Check sheet for the modelled part. Datum: model origin and axes. Units: mm. Round coordinates to 2 decimals unless told otherwise and drop trailing zeros. Write each loop counter-clockwise with the first axis right and the second up, starting at its lowest first coordinate (ties: lowest second). Pieces come first, ordered by that corner, then holes. Notation, with made-up numbers: (39, 74) -> (55, 74) arc R32 cw to (55, 109) -> close; hole circle Ø10 at (44, -31). An arc over 180 degrees is marked (long way). One line per item, written item: value.
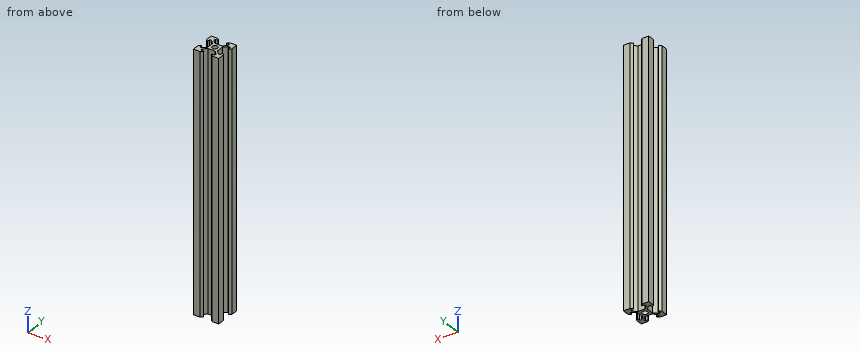
from build123d import *

# Parameters (mm, degrees)
SKETCH1_R           = 2.1
BOSS_EXTRUDE1_DEPTH = 200


with BuildPart() as part:
    # Sketch1 → Boss-Extrude1 (new body)
    with BuildSketch(Plane.XY):
        with BuildLine():
            Line((-2.839339828, 3.9), (-5.470710678, 6.53137085))
            ThreePointArc((-5.470710678, 6.53137085), (-5.492387953, 6.563813185), (-5.5, 6.602081528))
            Line((-5.5, 6.602081528), (-5.5, 8.1))
            ThreePointArc((-5.5, 8.1), (-5.470710678, 8.170710678), (-5.4, 8.2))
            Line((-5.4, 8.2), (-3.334418044, 8.2))
            ThreePointArc((-3.334418044, 8.2), (-3.244178397, 8.256909326), (-3.2566483, 8.362863876))
            Line((-3.2566483, 8.362863876), (-4.58, 10))
            Line((-4.58, 10), (-10, 10))
            Line((-10, 10), (-10, 4.58))
            Line((-10, 4.58), (-8.362863876, 3.2566483))
            ThreePointArc((-8.362863876, 3.2566483), (-8.256909326, 3.244178397), (-8.2, 3.334418044))
            Line((-8.2, 3.334418044), (-8.2, 5.4))
            ThreePointArc((-8.2, 5.4), (-8.170710678, 5.470710678), (-8.1, 5.5))
            Line((-8.1, 5.5), (-6.602081528, 5.5))
            ThreePointArc((-6.602081528, 5.5), (-6.563813185, 5.492387953), (-6.53137085, 5.470710678))
            Line((-6.53137085, 5.470710678), (-3.9, 2.839339828))
            Line((-3.9, 2.839339828), (-3.9, -2.839339828))
            Line((-3.9, -2.839339828), (-6.53137085, -5.470710678))
            ThreePointArc((-6.53137085, -5.470710678), (-6.563813185, -5.492387953), (-6.602081528, -5.5))
            Line((-6.602081528, -5.5), (-8.1, -5.5))
            ThreePointArc((-8.1, -5.5), (-8.170710678, -5.470710678), (-8.2, -5.4))
            Line((-8.2, -5.4), (-8.2, -3.334418044))
            ThreePointArc((-8.2, -3.334418044), (-8.256909326, -3.244178397), (-8.362863876, -3.2566483))
            Line((-8.362863876, -3.2566483), (-10, -4.58))
            Line((-10, -4.58), (-10, -10))
            Line((-10, -10), (-4.58, -10))
            Line((-4.58, -10), (-3.2566483, -8.362863876))
            ThreePointArc((-3.2566483, -8.362863876), (-3.244178397, -8.256909326), (-3.334418044, -8.2))
            Line((-3.334418044, -8.2), (-5.4, -8.2))
            ThreePointArc((-5.4, -8.2), (-5.470710678, -8.170710678), (-5.5, -8.1))
            Line((-5.5, -8.1), (-5.5, -6.602081528))
            ThreePointArc((-5.5, -6.602081528), (-5.492387953, -6.563813185), (-5.470710678, -6.53137085))
            Line((-5.470710678, -6.53137085), (-2.839339828, -3.9))
            Line((-2.839339828, -3.9), (2.839339828, -3.9))
            Line((2.839339828, -3.9), (5.470710678, -6.53137085))
            ThreePointArc((5.470710678, -6.53137085), (5.492387953, -6.563813185), (5.5, -6.602081528))
            Line((5.5, -6.602081528), (5.5, -8.1))
            ThreePointArc((5.5, -8.1), (5.470710678, -8.170710678), (5.4, -8.2))
            Line((5.4, -8.2), (3.334418044, -8.2))
            ThreePointArc((3.334418044, -8.2), (3.244178397, -8.256909326), (3.2566483, -8.362863876))
            Line((3.2566483, -8.362863876), (4.58, -10))
            Line((4.58, -10), (10, -10))
            Line((10, -10), (10, -4.58))
            Line((10, -4.58), (8.362863876, -3.2566483))
            ThreePointArc((8.362863876, -3.2566483), (8.256909326, -3.244178397), (8.2, -3.334418044))
            Line((8.2, -3.334418044), (8.2, -5.4))
            ThreePointArc((8.2, -5.4), (8.170710678, -5.470710678), (8.1, -5.5))
            Line((8.1, -5.5), (6.602081528, -5.5))
            ThreePointArc((6.602081528, -5.5), (6.563813185, -5.492387953), (6.53137085, -5.470710678))
            Line((6.53137085, -5.470710678), (3.9, -2.839339828))
            Line((3.9, -2.839339828), (3.9, 2.839339828))
            Line((3.9, 2.839339828), (6.53137085, 5.470710678))
            ThreePointArc((6.53137085, 5.470710678), (6.563813185, 5.492387953), (6.602081528, 5.5))
            Line((6.602081528, 5.5), (8.1, 5.5))
            ThreePointArc((8.1, 5.5), (8.170710678, 5.470710678), (8.2, 5.4))
            Line((8.2, 5.4), (8.2, 3.334418044))
            ThreePointArc((8.2, 3.334418044), (8.256909326, 3.244178397), (8.362863876, 3.2566483))
            Line((8.362863876, 3.2566483), (10, 4.58))
            Line((10, 4.58), (10, 10))
            Line((10, 10), (4.58, 10))
            Line((4.58, 10), (3.2566483, 8.362863876))
            ThreePointArc((3.2566483, 8.362863876), (3.244178397, 8.256909326), (3.334418044, 8.2))
            Line((3.334418044, 8.2), (5.4, 8.2))
            ThreePointArc((5.4, 8.2), (5.470710678, 8.170710678), (5.5, 8.1))
            Line((5.5, 8.1), (5.5, 6.602081528))
            ThreePointArc((5.5, 6.602081528), (5.492387953, 6.563813185), (5.470710678, 6.53137085))
            Line((5.470710678, 6.53137085), (2.839339828, 3.9))
            Line((2.839339828, 3.9), (-2.839339828, 3.9))
        make_face()
        Circle(SKETCH1_R, mode=Mode.SUBTRACT)
    extrude(amount=BOSS_EXTRUDE1_DEPTH)


solid = part.part
Item 1: Sectioned sample at A-A (x = 0). Enter the section's corners in (y, z).
Result set:
outline: (-3.9, 0) -> (-2.1, 0) -> (-2.1, 200) -> (-3.9, 200) -> close; (2.1, 0) -> (3.9, 0) -> (3.9, 200) -> (2.1, 200) -> close
Item 2: Depth check by flat-ended pin: pin 1 (5 mm diameter, centred on x = 0, y = 0, fed in from +Z); pin 2 (3 mm diameter, centred on x = 1, z = 118.5, fed in from -Y); pin 3 (6 mm diameter, centred on x = -1, z = 117, fed in from +Y); pin 4 (1.7 mm diameter, centred on y = 1, z = 79, fed in from +X). Enter the tip coordinate at first touch or a pass-through.
Result set:
pin 1: z = 200
pin 2: y = -3.9
pin 3: y = 9.28
pin 4: x = 3.9
Item 3: Material ranges on line 1 along Y through (x, z) = (0, 160.5); line 2 along Y through (x, z) = (-8.25, 169); line 3 along X through (y, z) = (-5, 160.5), recorded low to high.
Result set:
line 1: -3.9 to -2.1, 2.1 to 3.9
line 2: -10 to -3.25, 3.25 to 10
line 3: -10 to -8.2, -6.06 to -3.94, 3.94 to 6.06, 8.2 to 10
